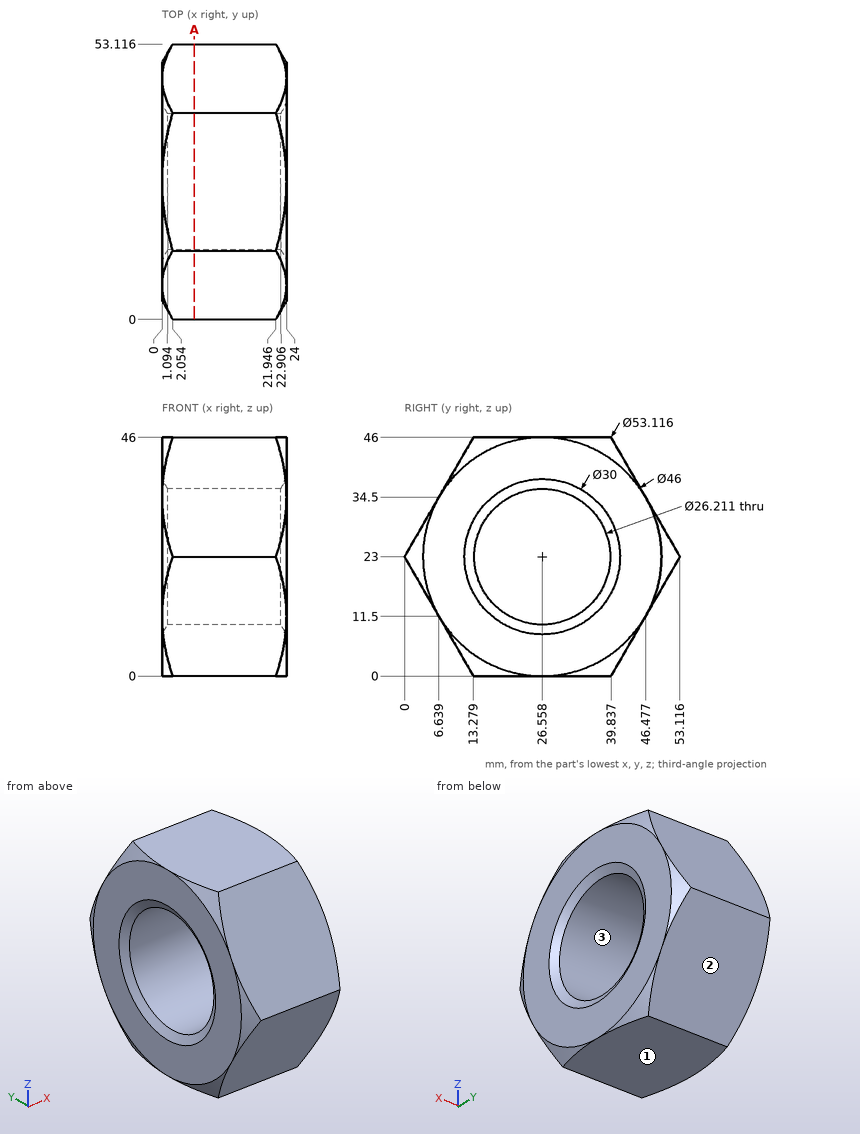
Print and shaded views of the part. All mm, measured from the part's lowest x, y and z. Round coordinates to 2 decimals unless told otherwise and drop trailing zeros. Write each loop counter-clockwise with the first axis right and the second up, starting at its lowest first coordinate (ties: lowest second). Pieces come first, ordered by that corner, then holes. Notation, with made-up numbers: (32.25, 66) -> (43.25, 66) arc R8 cw to (43.25, 70) -> close; hole circle Ø5 at (1, 39.5). An arc over 180 degrees is marked (long way). Return JSON: item names as keys, results as strings. Group by question number.
Q1. Probe L1, parallel to Y at x = 20.75, z = 23 (1 decimal); L2, parallel to Y at x = 16, z = 19 (1 decimal); L3, parallel to Z at x = 16.75, y = 36. List the from-to ranges inside material, lowest first. Write a range as [from, to].
Q2. Mould opens along Y. For the marked faces 1, 2 and 3 say: pulls with the +Y half, pulls with the -Y half, needs draft (parallel to the pull), parting line crosses it, or undercut.
Q3. Pin check, flat tip, straight feed: pin 1 (4 mm diameter, centred on x = 19.5, z = 15, fed in from -Y) (1 decimal). Stop position of the tip, or through.
Q4. Saw through at A-A on x = 6.25. Write the cut outline in (y, z) (1 decimal), plus the area to 3 significant figures.
Answer:
{
 "1": {"L1": "[0, 13.5], [39.7, 53.1]", "L2": "[2.3, 14.1], [39, 50.8]", "L3": "[0, 13.91], [32.09, 46]"},
 "2": {"face 1": "needs draft", "face 2": "pulls with the +Y half", "face 3": "undercut"},
 "3": {"pin 1": "y = 3.5"},
 "4": {"outline": "(0, 23) -> (13.3, 0) -> (39.8, 0) -> (53.1, 23) -> (39.8, 46) -> (13.3, 46) -> close; hole circle Ø26.2 at (26.6, 23)", "area": "1,290 mm2"}
}
